Geometry: see drawing. Coordinates: mm, zero at the bounding-box minimum. Give positions to 0.01 mm unless a question says otherwise; leave off trailing zeros. Write each loop counter-clockwise with the first axis right and the second up, starting at its lowest first coordinate (ties: lowest second). Pieces come first, ordered by that corner, then holes. Notation, with made-up numbers: (72, 22.25) - (117, 22.25) arc R33 cw to (117, 51.25) - close; hole circle Ø9 at (39.5, 65). An arc over 180 degrees is marked (long way). Return JSON: item names as keys, results as strings.
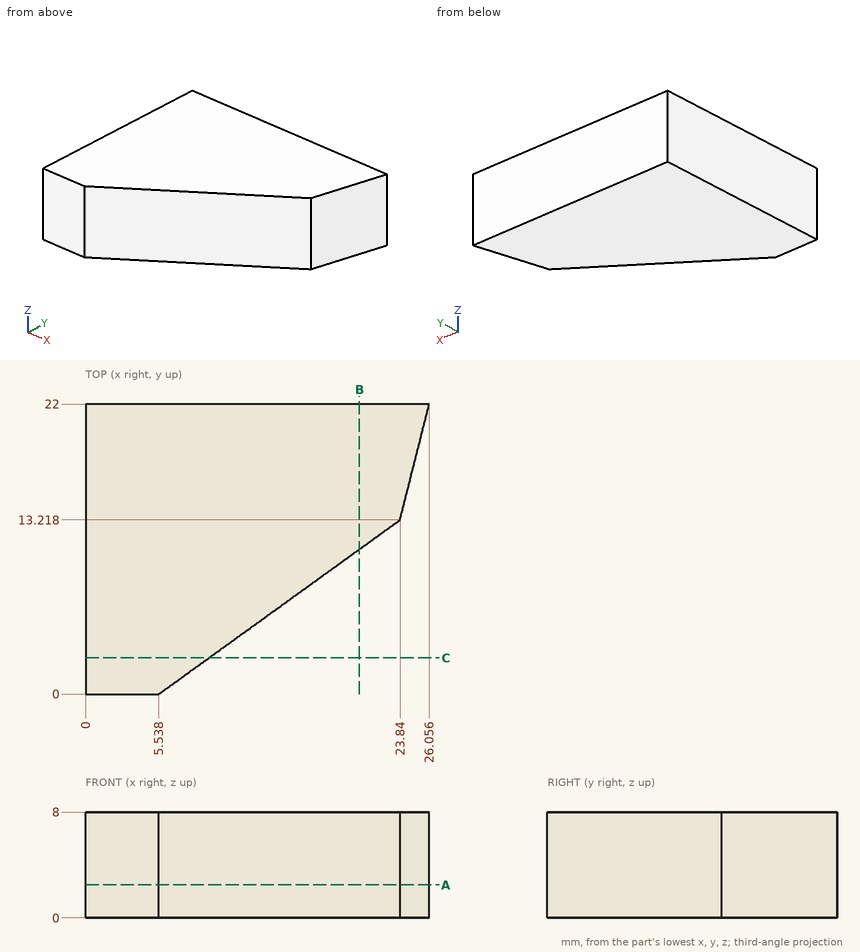
Q1. Section query B-B, the plane x = 20.75. Return the cut outline in (y, z), plus the area to 3 significant figures.
Answer key:
{"outline": "(10.99, 0) - (22, 0) - (22, 8) - (10.99, 8) - close", "area": "88.1 mm^2"}
Q2. Section query C-C, the plane y = 2.75. Return the cut outline in (x, z).
Answer key:
{"outline": "(0, 0) - (9.35, 0) - (9.35, 8) - (0, 8) - close"}
Q3. Section query A-A, the plane z = 2.5. Return the cut outline in (x, y).
Answer key:
{"outline": "(0, 0) - (5.54, 0) - (23.84, 13.22) - (26.06, 22) - (0, 22) - close"}
Q4. Material intervals for probe 1 along Y at (x, z) = (10.25, 7.25) (1 decimal); probe 2 along Y at (x, z) = (23.5, 2.25); probe 3 along X at (y, z) = (3, 3.25) (1 decimal), sorted ascending. Write a range as [from, to].
Answer key:
{"probe 1": "y = [3.4, 22]", "probe 2": "y = [12.97, 22]", "probe 3": "x = [0, 9.7]"}
